Check sheet for the drawn part. Datum: minimum x, y, z corner. Units: mm. Give positions to 0.01 mm unless a question says otherwise; leave off trailing zeros. Loops run counter-clockwise (first coordinate to the right, second up) from the corner with the lowest first, then second, coordinate; pieces in that order, holes last.
1. Cross-section at D-D, the plane y = 13.25. Record the cut outline in (x, z), plus the area to 3 significant figures.
2. Cross-section at A-A, the plane x = 15. Record the cut outline in (y, z).
3. Go/stop test with a flat-tipped pin: pin 1 Ø3 at (y, z) = (15, 8.5) entering from -X. Record where the tip stops, or that it passes through.
4. Release check for a two-part mould opening along Z. For the marked faces 1, 2, 3 and 4 record: +Z half, -Z half, draft (parallel to the pull), parting line (faces both ways), or undercut.
5. Cross-section at C-C, the plane z = 7.5. Record the cut outline in (x, y).
6. Cross-section at B-B, the plane y = 28.25. Record the cut outline in (x, z).
7. Material ranges on L1, parallel to Z at x = 15, y = 10.25; L2, parallel to X at y = 15.25, z = 7.5; L3, parallel to X at y = 26.55, z = 7.5, recorded low to high.
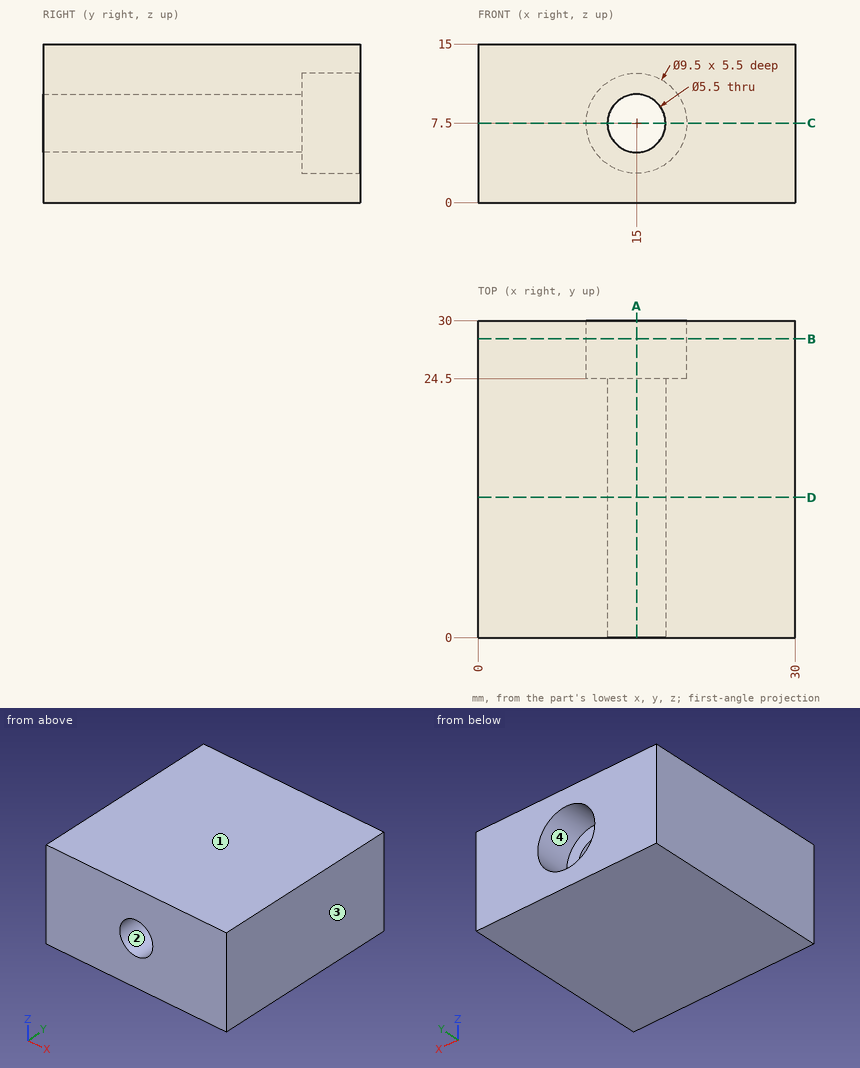
Result:
1. outline: (0, 0) - (30, 0) - (30, 15) - (0, 15) - close; hole circle Ø5.5 at (15, 7.5)
1. area: 426 mm2
2. outline: (0, 0) - (30, 0) - (30, 2.75) - (24.5, 2.75) - (24.5, 4.75) - (0, 4.75) - close; (0, 10.25) - (24.5, 10.25) - (24.5, 12.25) - (30, 12.25) - (30, 15) - (0, 15) - close
3. pin 1: stops at x = 0
4. face 1: +Z half
4. face 2: undercut
4. face 3: draft
4. face 4: undercut
5. outline: (0, 0) - (12.25, 0) - (12.25, 24.5) - (10.25, 24.5) - (10.25, 30) - (0, 30) - close; (17.75, 0) - (30, 0) - (30, 30) - (19.75, 30) - (19.75, 24.5) - (17.75, 24.5) - close
6. outline: (0, 0) - (30, 0) - (30, 15) - (0, 15) - close; hole circle Ø9.5 at (15, 7.5)
7. L1: z = 0 to 4.75, 10.25 to 15
7. L2: x = 0 to 12.25, 17.75 to 30
7. L3: x = 0 to 10.25, 19.75 to 30
